from build123d import *

# Parameters (mm, degrees)
SKETCH_1_W          = 24.7
SKETCH_1_H          = 24.7
SKETCH_1_W_2        = 12.7
SKETCH_1_H_2        = 12.7
EXTRUDE_2_DEPTH     = 24.7
EXTRUDE_3_DEPTH     = 14
EXTRUDE_4_DEPTH     = 14
SKETCH_5_R          = 2.5
CUT_EXTRUDE_1_DEPTH = 49.420398594
SKETCH_6_R          = 2.5
CUT_EXTRUDE_2_DEPTH = 48.542638757


with BuildPart() as part:
    # 草图1 → 凸台-拉伸2 (new body)
    # profile 1 of 2: a face of its own
    with BuildSketch(Plane(origin=(0, 0, 0), x_dir=(1, 0, 0), z_dir=(0, 1, 0))):
        Rectangle(SKETCH_1_W, SKETCH_1_H)
        Rectangle(SKETCH_1_W_2, SKETCH_1_H_2, mode=Mode.SUBTRACT)
    # profile 2 of 2: a face of its own
    with BuildSketch(Plane(origin=(0, 0, 0), x_dir=(1, 0, 0), z_dir=(0, 1, 0))):
        Rectangle(SKETCH_1_W_2, SKETCH_1_H_2)
    extrude(amount=EXTRUDE_2_DEPTH)

    # 草图3 → 凸台-拉伸3 (add)
    with BuildSketch(Plane.XZ):
        Polygon((-6.35, 12.35), (-6.35, 6.35), (6.35, 6.35), (6.35, -6.35), (-6.35, -6.35), (-6.35, -12.35), (12.35, -12.35), (12.35, 12.35), align=None)
    extrude(amount=EXTRUDE_3_DEPTH)

    # 草图4 → 凸台-拉伸4 (add)
    with BuildSketch(Plane(origin=(0, 0, -12.35), x_dir=(-1, 0, 0), z_dir=(0, 0, -1))):
        Polygon((6.35, 6), (-6.35, 6), (-6.35, 18.7), (6.35, 18.7), (6.35, 24.7), (-12.35, 24.7), (-12.35, 0), (6.35, 0), align=None)
    extrude(amount=EXTRUDE_4_DEPTH)

    # 草图5 → 切除-拉伸1 (cut, through all)
    with BuildSketch(Plane(origin=(0, 24.7, 0), x_dir=(1, 0, 0), z_dir=(0, 1, 0))):
        with Locations(Location((0, 19.98, 0), (0, 0, 270))):
            Circle(SKETCH_5_R)
    extrude(amount=-CUT_EXTRUDE_1_DEPTH, mode=Mode.SUBTRACT)

    # 草图6 → 切除-拉伸2 (cut, through all)
    with BuildSketch(Plane.XY.offset(12.35)):
        with Locations((0, -7.63)):
            Circle(SKETCH_6_R)
    extrude(amount=-CUT_EXTRUDE_2_DEPTH, mode=Mode.SUBTRACT)


solid = part.part
Here's how the part is built. I have some questions about the finished solid (model axes, mm). A direction names the side the tool comes from. Coordinates: 2 decimals unless noted, no trailing zeros. Write each loop counter-clockwise with the first axis right and the second up, starting at its lowest first coordinate (ties: lowest second). Pieces come first, ordered by that corner, then holes.
1) Thinking about a two-plate mould opening in Y: for faces 5 (the face through (-0.54, -10.07, 9.39)), 6 (the face through (0.751, 3.042, -17.595)), 7 (the face through (3, 0, -19)), which applies, +Y half, -Y half, draft (parallel to the pull), parting line (faces both ways), or undercut?
Filled in:
face 5: undercut
face 6: draft
face 7: -Y half
2) If we section it at A-A (z = -10.5): List the corners of the cut face in (x, y) for me, plus the area to 3 significant figures.
Filled in:
outline: (-12.35, 0) - (-6.35, 0) - (-6.35, -14) - (12.35, -14) - (12.35, 24.7) - (-12.35, 24.7) - close; hole circle Ø5 at (0, -7.63)
area: 852 mm2
3) I'm going to push flat-ended pins straight in: pin 1 (4 mm diameter, centred on x = 0, y = -7.63, fed in from +Z); pin 2 (6 mm diameter, centred on x = 0, z = -19.98, fed in from -Y); pin 3 (1.5 mm diameter, centred on y = 14.5, z = -18.5, fed in from -X); pin 4 (4 mm diameter, centred on x = -3, y = -5.5, fed in from -Z). Where does each tip first touch, or does it pass through?
Filled in:
pin 1: passes through
pin 2: stops at y = 0
pin 3: stops at x = 6.35
pin 4: stops at z = -12.35
4) If we section it at D-D (z = -19.98): List the corners of the cut face in (x, y) for me, plus the area to 3 significant figures.
Filled in:
outline: (-6.35, 0) - (-2.5, 0) - (-2.5, 6) - (-6.35, 6) - close; (-6.35, 18.7) - (-2.5, 18.7) - (-2.5, 24.7) - (-6.35, 24.7) - close; (2.5, 0) - (12.35, 0) - (12.35, 24.7) - (2.5, 24.7) - (2.5, 18.7) - (6.35, 18.7) - (6.35, 6) - (2.5, 6) - close
area: 241 mm2
5) If we section it at B-B (y = -7.63): List the corners of the cut face in (x, z) for me, plus the area to 3 significant figures.
Filled in:
outline: (-6.35, -12.35) - (-2.5, -12.35) - (-2.5, -6.35) - (-6.35, -6.35) - close; (-6.35, 6.35) - (-2.5, 6.35) - (-2.5, 12.35) - (-6.35, 12.35) - close; (2.5, -12.35) - (12.35, -12.35) - (12.35, 12.35) - (2.5, 12.35) - (2.5, 6.35) - (6.35, 6.35) - (6.35, -6.35) - (2.5, -6.35) - close
area: 241 mm2
6) Which directions (+Z, -Z, +X, -X, +Y, -Y) give clear straight access to the entire face, cutting with the end or side of a thin tool? Please do faces 1 (the face through (-6.35, 3, -19)), 2 (the face through (2, 18.7, -18)), 3 (the face through (-6.35, -7, -9)), 4 (the face through (-1, -5, -6.35)).
Filled in:
face 1: -Z, -X, +Y, -Y
face 2: -Z, -X
face 3: +Z, -Z, -X, -Y
face 4: -X, -Y
7) If we section it at C-C (x = 0): Count the separate pieces of the cut face and the enclosed holes in it, plus the area to 3 significant figures.
Filled in:
separate pieces: 5
enclosed holes: 0
area: 826 mm2
8) If I drill on line 1 (Y direction, x = 0, z = -11); line 2 (Y direction, x = -1, z = -23); line 3 (Z direction, x = -5, y = -8.5), over which ranges is the centre line in solid material (lowest first)?
Filled in:
line 1: y = -14 to -10.13, -5.13 to 24.7
line 2: y = 0 to 6, 18.7 to 24.7
line 3: z = -12.35 to -6.35, 6.35 to 12.35
